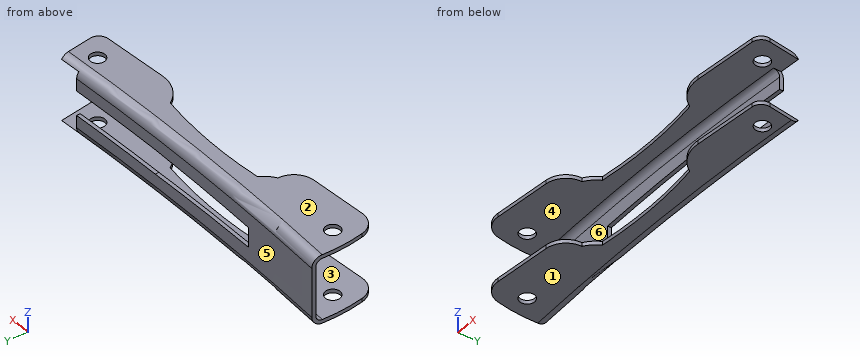
from build123d import *

# Parameters (mm, degrees)
BOSS_EXTRUDE1_DEPTH = 7
FILLET1_R           = 4
FILLET2_R           = 2
SHELL1_T            = -0.75
CUT_EXTRUDE1_DEPTH  = 14
SKETCH5_R           = 1.5
CUT_EXTRUDE2_DEPTH  = 71.716642035
CUT_EXTRUDE3_DEPTH  = 71.716642035


with BuildPart() as part:
    # Sketch2 → Boss-Extrude1 (new, symmetric)
    with BuildSketch(Plane.XY):
        with BuildLine():
            Line((67, 0), (68.2, -9))
            Line((68.2, -9), (1.2, -14))
            Line((1.2, -14), (0, 0))
            ThreePointArc((0, 0), (33.5, -1), (67, 0))
        make_face()
        with BuildLine():
            ThreePointArc((1.2, -14), (-0.147259987, -7.064050856), (0, 0))
            Line((0, 0), (1.2, -14))
        make_face()
    extrude(amount=BOSS_EXTRUDE1_DEPTH, both=True)

    # Fillet1
    fillet1_edges = [part.edges().sort_by_distance(p)[0] for p in [
        (1.2, -14, 0),
    ]]
    fillet(fillet1_edges, radius=FILLET1_R)

    # Fillet2
    fillet2_edges = [part.edges().sort_by_distance(p)[0] for p in [
        (33.5, -1, 7),
        (33.5, -1, -7),
        (68.2, -9, 0),
    ]]
    fillet(fillet2_edges, radius=FILLET2_R)

    # Shell1
    shell1_openings = [part.faces().sort_by_distance(p)[0] for p in [
        (67.467137389, -3.50353042, 6e-09),
        (1.829469038, -12.937587905, 0),
        (67.490186671, -8.423793277, 0),
        (35.321845663, -11.453593607, 0),
        (-0.252281581, -5.271781297, 0),
    ]]
    offset(amount=SHELL1_T, openings=shell1_openings)

    # Sketch4 → Cut-Extrude1 (cut)
    with BuildSketch(Plane(origin=(0, 0, 0), x_dir=(1, 0, 0), z_dir=(0, 1, 0))):
        Polygon((17.8, -2), (17.8, 2), (42.8, 2.5), (62.8, 2.5), (62.8, 6.25), (67.8, 6.25), (67.8, -6.25), (62.8, -6.25), (62.8, -2.5), (42.8, -2.5), align=None)
    extrude(amount=-CUT_EXTRUDE1_DEPTH, mode=Mode.SUBTRACT)

    # Sketch5 → Cut-Extrude2 (cut, through all)
    with BuildSketch(Plane.XY.offset(7)):
        with Locations((3.95, -7.3)):
            Circle(SKETCH5_R)
        with Locations((63.108141066, -4.736057992)):
            Circle(SKETCH5_R)
    extrude(amount=-CUT_EXTRUDE2_DEPTH, mode=Mode.SUBTRACT)

    # Sketch6 → Cut-Extrude3 (cut, through all)
    with BuildSketch(Plane.XY.offset(7)):
        with BuildLine():
            Line((16.25, -12.876865672), (53, -10.134328358))
            ThreePointArc((53, -10.134328358), (49.280996353, -9.38144837), (46.5, -6.8))
            ThreePointArc((46.5, -6.8), (34.520096022, -5.696159139), (22.5, -6.2))
            ThreePointArc((22.5, -6.2), (21.525014111, -7.562463141), (20.229840096, -8.625208437))
            ThreePointArc((20.229840096, -8.625208437), (19.06924649, -11.527342961), (16.25, -12.876865672))
        make_face()
    extrude(amount=-CUT_EXTRUDE3_DEPTH, mode=Mode.SUBTRACT)


solid = part.part
Build history of the part. All positions in model axes, mm. Face numbers are marked on the shaded views. A direction names the side the tool comes from. Give positions to 0.01 mm unless a question says otherwise; leave off trailing zeros. Loops run counter-clockwise (first coordinate to the right, second up) from the corner with the lowest first, then second, coordinate; pieces in that order, holes last. Notation, with made-up numbers: (-36, 88.5) -> (21, 88.5) arc R38 ccw to (21, 127.5) -> close; hole circle Ø2 at (19.5, 34.5). An arc over 180 degrees is marked (long way). Answer in a Markdown table with one row per item.
Item 1: Tool access for the marked faces 5 and 6: list every direction of +Z, -Z, +X, -X, +Y, -Y with a clear straight run to the whole face (end or side of a thin tool).
Findings below:
| item | result |
|---|---|
| face 5 | +Z, -Z, +Y |
| face 6 | -Y |
Item 2: Mould opens along Z. For the marked faces 1, 2, 3 and 4 say: pulls with the +Z half, pulls with the -Z half, needs draft (parallel to the pull), parting line crosses it, or undercut.
Findings below:
| item | result |
|---|---|
| face 1 | pulls with the -Z half |
| face 2 | pulls with the +Z half |
| face 3 | undercut |
| face 4 | undercut |
Item 3: Slice it at A-A on y = -4. Write the cut outline in (x, z), plus the area to 3 significant figures.
Findings below:
| item | result |
|---|---|
| outline | (-0.27, -7) -> (61.8, -7) -> (61.8, -6.25) -> (-0.27, -6.25) -> close; (-0.27, 6.25) -> (61.8, 6.25) -> (61.8, 7) -> (-0.27, 7) -> close; (64.42, -7) -> (67.53, -7) -> (67.53, -6.25) -> (64.42, -6.25) -> close; (64.42, 6.25) -> (67.53, 6.25) -> (67.53, 7) -> (64.42, 7) -> close |
| area | 97.8 mm² |
Item 4: Flat gauge pins, fed straight in: P1, Ø1, axis at y = -1, z = 3.5, coming from the +X side; P2, Ø4, axis at y = -5.5, z = -2.5, coming from the +X side; P3, Ø2, axis at x = 41, z = 1.5, coming from the +Y side; P4, Ø1.6, axis at x = 57, y = -1, coming from the -Z side. Where does each tip first touch, or does it go through?
Findings below:
| item | result |
|---|---|
| P1 | stops at x = 62.8 |
| P2 | passes through |
| P3 | stops at y = -0.95 |
| P4 | stops at z = -6.87 |
Item 5: Slice it at D-D on x = 3.95. Give the number of separate pieces and of enclosed holes in the cut face, plus the area to 3 significant figures.
Findings below:
| item | result |
|---|---|
| separate pieces | 3 |
| enclosed holes | 0 |
| area | 24.1 mm² |
Item 6: Slice it at C-C on z = 0.5. Write the cut outline in (x, y) (3 decimals), plus the area to 3 significant figures.
Findings below:
| item | result |
|---|---|
| outline | (-0.087, -0.746) arc R562.375 ccw to (17.8, -1.531) -> (17.8, -0.781) arc R561.625 cw to (0, 0) arc R33.282 ccw to start |
| area | 13.4 mm² |
Item 7: Probe line 1 along Z through (x, y) = (11.5, -10); line 2 along Y through (x, z) = (3.95, -6.65). List the from-to ranges inside material, lowest first. Write a range as [from, to].
Findings below:
| item | result |
|---|---|
| line 1 | z = [-7, -6.25], [6.25, 7] |
| line 2 | y = [-13.75, -8.8], [-5.8, -1.09] |
Item 8: Slice it at B-B on y = -11.5. Write the cut outline in (x, z).
Findings below:
| item | result |
|---|---|
| outline | (0.66, -7) -> (19.09, -7) -> (19.09, -6.25) -> (0.66, -6.25) -> close; (0.66, 6.25) -> (19.09, 6.25) -> (19.09, 7) -> (0.66, 7) -> close |
